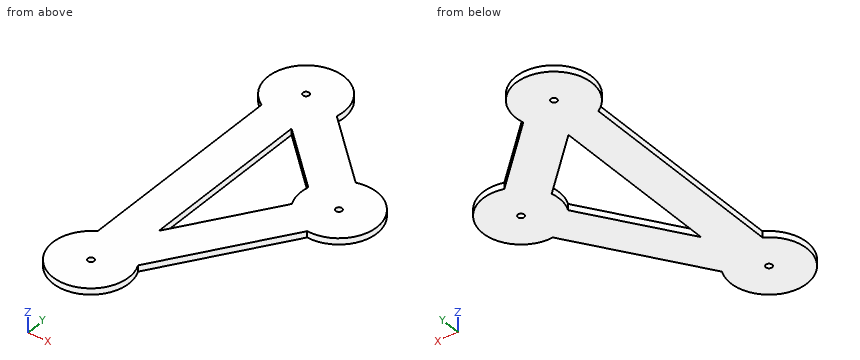
from build123d import *

# Parameters (mm, degrees)
SKETCH1_R           = 3.1115
BOSS_EXTRUDE1_DEPTH = 6.223


with BuildPart() as part:
    # Sketch1 → Boss-Extrude1 (new body)
    with BuildSketch(Plane.XY):
        with BuildLine():
            ThreePointArc((56.241862877, 269.861061996), (3.715941389, 313.008025267), (0, 245.134432116))
            Line((0, 245.134432116), (0, 32.995567884))
            ThreePointArc((0, 32.995567884), (8.068918145, -36.483226849), (53.14774846, 16.998633767))
            Line((53.14774846, 16.998633767), (131.266861023, 135.012436144))
            ThreePointArc((131.266861023, 135.012436144), (171.412005233, 177.672174614), (122.159665516, 209.384836474))
            Line((122.159665516, 209.384836474), (56.241862877, 269.861061996))
        make_face()
        with Locations((19.05, 0)):
            Circle(SKETCH1_R, mode=Mode.SUBTRACT)
        with Locations((19.05, 278.13)):
            Circle(SKETCH1_R, mode=Mode.SUBTRACT)
        with BuildLine():
            Line((99.496738121, 156.042635639), (38.1, 63.291165717))
            Line((38.1, 63.291165717), (38.1, 234.79989424))
            Line((38.1, 234.79989424), (96.402623704, 181.31020741))
            ThreePointArc((96.402623704, 181.31020741), (95.77696793, 168.410364199), (99.496738121, 156.042635639))
        make_face(mode=Mode.SUBTRACT)
        with Locations((133.594486582, 173.041269406)):
            Circle(SKETCH1_R, mode=Mode.SUBTRACT)
    extrude(amount=BOSS_EXTRUDE1_DEPTH)


solid = part.part
CAD build for the part. Positions are in the model's coordinates, mm. Coordinates: 2 decimals unless noted, no trailing zeros. Loops run counter-clockwise (first coordinate to the right, second up) from the corner with the lowest first, then second, coordinate; pieces in that order, holes last. Notation, with made-up numbers: (31, 33) -> (83, 33) arc R9 cw to (83, 39) -> close; hole circle Ø4 at (87, 54). An arc over 180 degrees is marked (long way). One line per item, written item: value.
1. Drill centre lines: line 1 (X direction, y = 278.13, z = 1.5); line 2 (X direction, y = 73, z = 0.5); line 3 (Y direction, x = -3.5, z = 4.25). Where is each one in solid material? Low to high. Write a range as [from, to].
Answers:
line 1: x = [-19.05, 15.94], [22.16, 57.15]
line 2: x = [0, 38.1], [44.53, 90.22]
line 3: y = [-30.71, 30.71], [247.42, 308.84]
2. Flat gauge pins, fed straight in: P1, Ø1, axis at y = 224.5, z = 4.5, coming from the -X side; P2, Ø3, axis at x = 5.5, z = 1.5, coming from the +Y side; P3, Ø1, axis at x = 27, z = 5, coming from the +Y side. Where does each tip first touch, or does it go through?
Answers:
P1: stops at x = 0
P2: stops at y = 314.27
P3: stops at y = 315.49
3. Slice it at B-B on x = 73.5. Write the cut outline in (y, z).
Answers:
outline: (47.74, 0) -> (116.77, 0) -> (116.77, 6.22) -> (47.74, 6.22) -> close; (202.32, 0) -> (254.03, 0) -> (254.03, 6.22) -> (202.32, 6.22) -> close
4. Slice it at C-C on z = 4. Write the cut outline in (x, y), and give its area (3 significant figures).
Answers:
outline: (0, 33) arc R38.1 ccw (long way) to (53.15, 17) -> (131.27, 135.01) arc R38.1 ccw (long way) to (122.16, 209.38) -> (56.24, 269.86) arc R38.1 ccw (long way) to (0, 245.13) -> close; hole circle Ø6.22 at (19.05, 0); hole circle Ø6.22 at (19.05, 278.13); hole (38.1, 63.29) -> (99.5, 156.04) arc R38.1 cw to (96.4, 181.31) -> (38.1, 234.8) -> close; hole circle Ø6.22 at (133.59, 173.04)
area: 29,400 mm^2
5. Slice it at D-D on x = 106.5. Write the cut outline in (y, z), and give its area (3 significant figures).
Answers:
outline: (97.6, 0) -> (223.75, 0) -> (223.75, 6.22) -> (97.6, 6.22) -> close
area: 785 mm^2
6. Slice it at A-A on y = 160.5. Write the cut outline in (x, z), and give its area (3 significant figures).
Answers:
outline: (0, 0) -> (38.1, 0) -> (38.1, 6.22) -> (0, 6.22) -> close; (97.62, 0) -> (169.57, 0) -> (169.57, 6.22) -> (97.62, 6.22) -> close
area: 685 mm^2
